Drawing for the job (mm, zero at the part's lowest x, y, z). Round coordinates to 2 decimals unless told otherwise and drop trailing zeros. Loops run counter-clockwise (first coordinate to the right, second up) from the corner with the lowest first, then second, coordinate; pieces in that order, holes last. Notation, with made-up numbers: M 26,35 L 42,35 A34 cw 42,69 Z; hole C 15.25,79 d9. An arc over 180 degrees is marked long. Use a Markdown table: item, result. Add a question column.
Q1. Cut at B-B (z = 43). Give the cut face in (x, y).
Q2. Probe line 1 (X direction, y = 0.75, z = 14); line 2 (Z direction, x = 31, y = 1.9); line 3 (X direction, y = 2.15, z = 49.5). List the from-to ranges inside material, lowest first. Write a range as from..to.
Q3. Cut at C-C (y = 0.9). State how many separate pieces and enclosed holes the cut face has, plus the area to 3 significant figures.
Q4. Cut at A-A (x = 26). Give the cut face in (y, z).
Q5. Pin check, flat tip, straight feed: pin 1 (0.9 mm diameter, centred on x = 29.5, y = 1, fed in from -Z). Stop position of the tip, or through.
Q6. Cut at D-D (x = 61). Give the cut face in (y, z), plus the area to 3 significant figures.
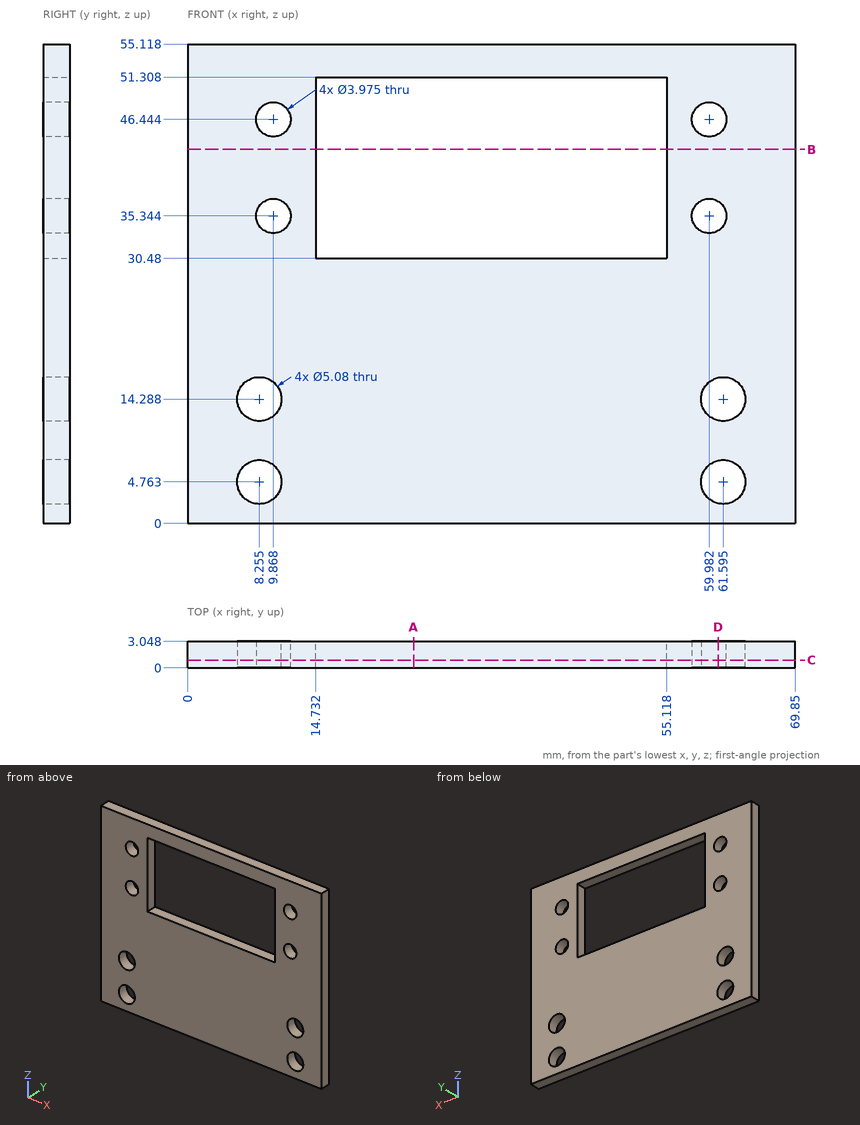
Checked values:
| question | item | result |
|---|---|---|
| 1 | outline | M 0,0 L 14.73,0 L 14.73,3.05 L 0,3.05 Z; M 55.12,0 L 69.85,0 L 69.85,3.05 L 55.12,3.05 Z |
| 2 | line 1 | x = 0..5.73, 10.78..59.07, 64.12..69.85 |
| 2 | line 2 | z = 0..30.48, 51.31..55.12 |
| 2 | line 3 | x = 0..14.73, 55.12..69.85 |
| 3 | separate pieces | 1 |
| 3 | enclosed holes | 9 |
| 3 | area | 2,880 mm^2 |
| 4 | outline | M 0,0 L 3.05,0 L 3.05,30.48 L 0,30.48 Z; M 0,51.31 L 3.05,51.31 L 3.05,55.12 L 0,55.12 Z |
| 5 | pin 1 | stops at z = 0 |
| 6 | outline | M 0,0 L 3.05,0 L 3.05,2.29 L 0,2.29 Z; M 0,7.23 L 3.05,7.23 L 3.05,11.82 L 0,11.82 Z; M 0,16.76 L 3.05,16.76 L 3.05,33.64 L 0,33.64 Z; M 0,37.05 L 3.05,37.05 L 3.05,44.74 L 0,44.74 Z; M 0,48.15 L 3.05,48.15 L 3.05,55.12 L 0,55.12 Z |
| 6 | area | 117 mm^2 |
